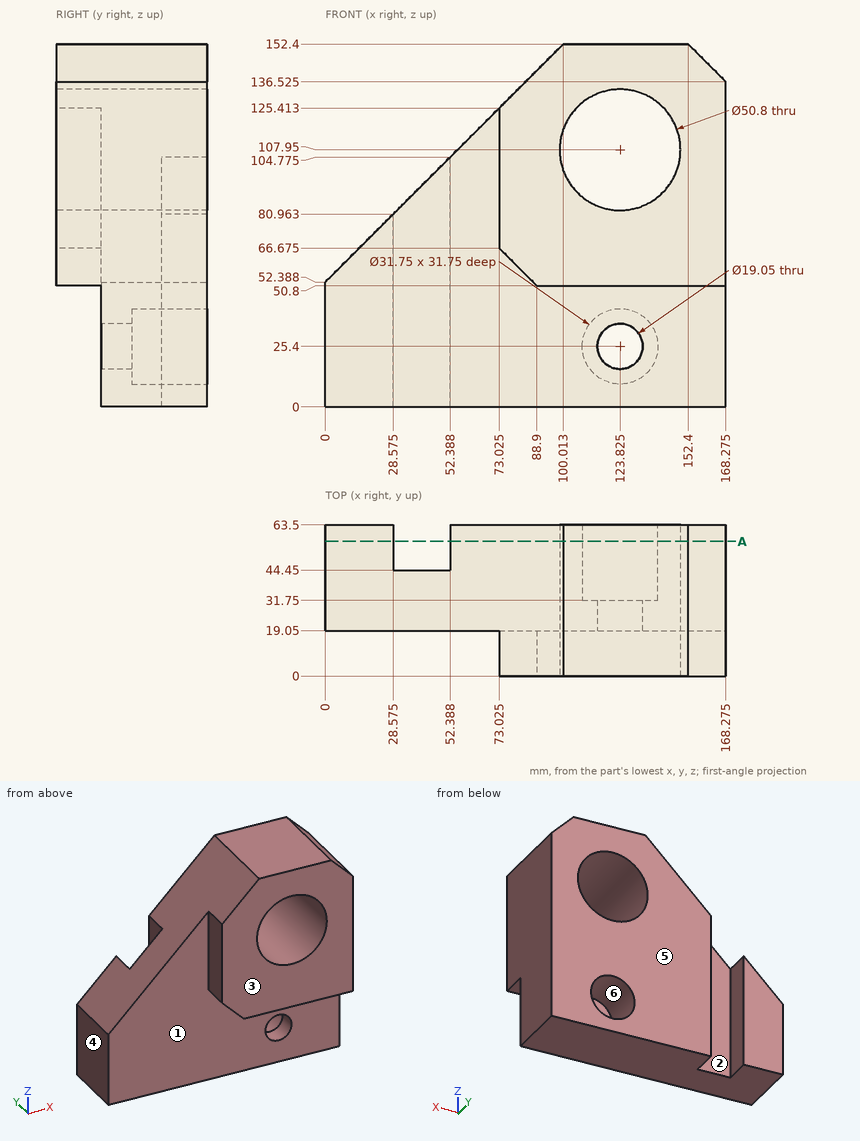
Can you work these out from the drawing? Everything is in mm from the part's minimum corner. A direction names the side the tool comes from. Coordinates: 2 decimals unless noted, no trailing zeros. One line per item, written item: value.
1) I need wall thicknesses on line 1 along X through (y, z) = (47.5, 15) (1 decimal); line 2 along Y through (x, z) = (39, 11.5); line 3 along Z through (x, y) = (131, 52.5) (1 decimal). Which ranges of each line are inside material? Lowest first, please.
Model answer:
line 1: x = 0 to 28.6, 52.4 to 111.8, 135.8 to 168.3
line 2: y = 19.05 to 44.45
line 3: z = 0 to 11.2, 39.6 to 83.6, 132.3 to 152.4
2) Suppose I cut it at A-A on y = 56.5. State how many separate pieces and enclosed holes the cut face has, and give its area (3 significant figures).
Model answer:
separate pieces: 2
enclosed holes: 2
area: 15,500 mm²
3) I'm going to push flat-ended pins straight in: P1, Ø3, axis at x = 137, z = 46.5, coming from the -Y side; P2, Ø21, axis at x = 143.5, y = 7, coming from the -Z side; P3, Ø1.5, axis at y = 28, z = 111.5, coming from the -X side. Where does each tip first touch, or does it pass through?
Model answer:
P1: stops at y = 19.05
P2: stops at z = 50.8
P3: stops at x = 58.36
4) On a 3-axis mill with a long thin cutter (end or side, diameter ignored), from which of +Z, -Z, +X, -X, +Y, -Y can I reach the whole of each face in a straight line? I mean the marked faces 1, 2 and 3. Say none if no direction works.
Model answer:
face 1: -Z, -X, -Y
face 2: +Z, -Z, +Y
face 3: +Z, -Z, +X, -X, -Y
5) We'd pull the mould along X, two halves only. Please class the marked faces 4, 5 and 6: pulls with the +X half, pulls with the -X half, needs draft (parallel to the pull), parting line crosses it, or undercut.
Model answer:
face 4: pulls with the -X half
face 5: needs draft
face 6: undercut
